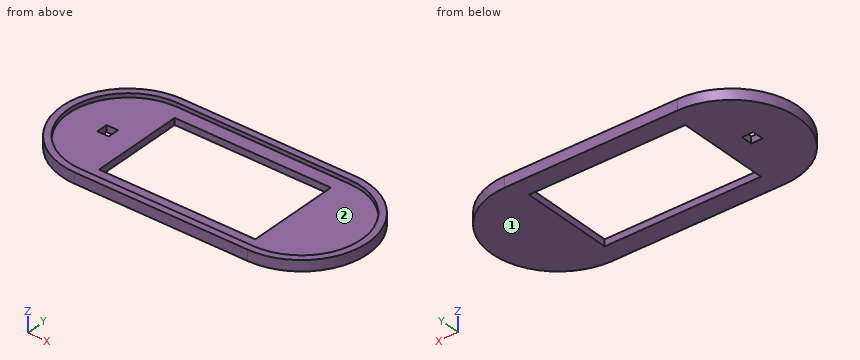
from build123d import *

# Parameters (mm, degrees)
BOSS_EXTRUDE1_DEPTH = 8
SHELL1_T            = -5
SKETCH2_W           = 117.4
SKETCH2_H           = 70.3
SKETCH2_W_2         = 8.6
SKETCH2_H_2         = 8.6
CUT_EXTRUDE1_DEPTH  = 5


with BuildPart() as part:
    # Sketch1 → Boss-Extrude1 (new body)
    with BuildSketch(Plane.XY):
        with BuildLine():
            Line((0, 0), (-130, 0))
            ThreePointArc((-130, 0), (-180, -50), (-130, -100))
            Line((-130, -100), (0, -100))
            ThreePointArc((0, -100), (50, -50), (0, 0))
        make_face()
    extrude(amount=BOSS_EXTRUDE1_DEPTH)

    # Shell1
    shell1_openings = [part.faces().sort_by_distance(p)[0] for p in [
        (-65, -50, 8),
    ]]
    offset(amount=SHELL1_T, openings=shell1_openings, kind=Kind.INTERSECTION)

    # Sketch2 → Cut-Extrude1 (cut)
    with BuildSketch(Plane(origin=(0, 0, 0), x_dir=(-1, 0, 0), z_dir=(0, 0, -1))):
        with Locations((65, -50)):
            Rectangle(SKETCH2_W, SKETCH2_H)
        with Locations((145.596085379, -50)):
            Rectangle(SKETCH2_W_2, SKETCH2_H_2)
    extrude(amount=-CUT_EXTRUDE1_DEPTH, mode=Mode.SUBTRACT)


solid = part.part
CAD build for the part. Positions are in the model's coordinates, mm. Face numbers are marked on the shaded views. Round coordinates to 2 decimals unless told otherwise and drop trailing zeros. Loops run counter-clockwise (first coordinate to the right, second up) from the corner with the lowest first, then second, coordinate; pieces in that order, holes last. Notation, with made-up numbers: M 83,9.25 L 136,9.25 A25 ccw 136,46.25 Z; hole C -8.75,-35.75 d7. An arc over 180 degrees is marked long. One line per question, with ' | ' between items. Start each with the question number.
Item 1: Wall check: line 1 (X direction, y = -50.5, z = 3.5); line 2 (Y direction, x = -55, z = 6.25); line 3 (Y direction, x = -117.5, z = 2.5). Give the ranges that are in metal, low to high.
Item 2: Cut at D-D, the plane y = -26. Write the cut outline in (x, z), plus the area to 3 significant figures.
Item 3: Pin check, flat tips, straight feed: pin 1 Ø4 at (y, z) = (-37, 7) entering from -X (3 decimals); pin 2 Ø1.5 at (y, z) = (-40.5, 2) entering from -X; pin 3 Ø4 at (x, z) = (-146.5, 2) entering from -Y. Stop position of each tip, or through.
Item 4: Cut at C-C, the plane z = 2.25. Write the cut outline in (x, y).
Item 5: Cut at A-A, the plane x = -91. Write the cut outline in (y, z), plus the area to 4 significant figures.
Item 6: Cut at B-B, the plane y = -50. Write the cut outline in (x, z), plus the area to 3 significant figures.
Item 7: Two-plate mould, pull along Y, no slides. Class the marked faces 1 and 2: pulls with the +Y half, pulls with the -Y half, needs draft (parallel to the pull), parting line crosses it, or undercut.
Responses:
1) line 1: x = -180 to -149.9, -141.3 to -123.7, -6.3 to 50 | line 2: y = -100 to -95, -5 to 0 | line 3: y = -100 to -85.15, -14.85 to 0
2) outline: M -173.86,0 L -123.7,0 L -123.7,5 L -168.07,5 L -168.07,8 L -173.86,8 Z; M -6.3,0 L 43.86,0 L 43.86,8 L 38.07,8 L 38.07,5 L -6.3,5 Z | area: 536 mm²
3) pin 1: stops at x = -178.775 | pin 2: stops at x = -179.23 | pin 3: stops at y = -97.85
4) outline: M -130,-100 L 0,-100 A50 ccw 0,0 L -130,0 A50 ccw Z; hole M -149.9,-54.3 L -141.3,-54.3 L -141.3,-45.7 L -149.9,-45.7 Z; hole M -123.7,-85.15 L -6.3,-85.15 L -6.3,-14.85 L -123.7,-14.85 Z
5) outline: M -100,0 L -85.15,0 L -85.15,5 L -95,5 L -95,8 L -100,8 Z; M -14.85,0 L 0,0 L 0,8 L -5,8 L -5,5 L -14.85,5 Z | area: 178.5 mm²
6) outline: M -180,0 L -149.9,0 L -149.9,5 L -175,5 L -175,8 L -180,8 Z; M -141.3,0 L -123.7,0 L -123.7,5 L -141.3,5 Z; M -6.3,0 L 50,0 L 50,8 L 45,8 L 45,5 L -6.3,5 Z | area: 550 mm²
7) face 1: needs draft | face 2: undercut
